Could you check a few things on this model? Use its own coordinates, in mm. A direction names the side the tool comes from. Coordinates: 2 decimals unless noted, no trailing zeros. Write each loop counter-clockwise with the first axis right and the second up, starting at its lowest first coordinate (ties: lowest second). Pieces come first, ordered by that corner, then holes. Notation, with made-up numbers: M -28,12.25 L -4,12.25 A12 ccw -4,16.25 Z; hole C 48,39.25 d11. An arc over 180 degrees is marked long. Answer as CSV lines item,"result". Start each with the question number.
Item 1: Suppose I cut it at B-B, the plane x = 0.25. Write out the boundary of the cut face in (y, z), and give its area (3 significant figures).
Item 2: We'd pull the mould along X, two halves only. Please class faces 5 (the flat face through (-2.74, -4, 3)), 6 (the flat face through (-6.584, -11, 4)), 7 (the flat face through (-9, -15, 2)), 8 (the flat face through (8.461, -4, 3)): +X half, -X half, draft (parallel to the pull), parting line (faces both ways), or undercut.
Item 3: On a 3-axis mill with a long thin cutter (end or side, diameter ignored), from which of +Z, -Z, +X, -X, +Y, -Y can I reach the whole of each face in a straight line? I mean faces 1 (the flat face through (3, -4, 4)), 2 (the flat face through (-9, -3.903, 5)), 3 (the flat face through (-9, -5.903, 4)), 4 (the flat face through (-2, -10.903, 1)). Say none if no direction works.
Item 4: Suppose I cut it at C-C, the plane z = 4.5. Write out the boundary of the cut face in (x, y), and give its area (3 significant figures).
Item 5: I'm going to push flat-ended pins straight in: P1, Ø7, axis at x = 2, y = -3, coming from the +Z side; P2, Ø1.6, axis at x = 5, z = 2.5, coming from the -Y side; P3, Ø2.5, axis at y = -13, z = 4.5, coming from the -X side. Where does each tip first touch, or does it pass through?
Item 6: Suppose I cut it at D-D, the plane x = -10. Write out the boundary of the cut face in (y, z).
Item 7: Suppose I cut it at A-A, the plane y = -12.25. Write out the boundary of the cut face in (x, z).
Item 8: If I drill on line 1 along Z through (x, y) = (7.25, -1); line 2 along Z through (x, y) = (-2.25, 1.75); line 3 along X through (y, z) = (-7.25, 5.25), over which ranges is the centre line in solid material (lowest first)? Write a range as [from, to].
```python
from build123d import *

# Parameters (mm, degrees)
SKETCH_2_W      = 25
SKETCH_2_H      = 15
EXTRUDE_1_DEPTH = 2
SKETCH_4_R      = 1.75
EXTRUDE_2_DEPTH = 7
SKETCH_5_W      = 5
SKETCH_5_H      = 5
EXTRUDE_3_DEPTH = 2
SKETCH_4_3_R    = 1.75
EXTRUDE_4_DEPTH = 2
SKETCH_7_W      = 11.201035141
SKETCH_7_H      = 8.645905099
EXTRUDE_5_DEPTH = 2
SKETCH_4_4_R    = 1.75
EXTRUDE_6_DEPTH = 8


with BuildPart() as part:
    # Sketch 2 → Extrude 1 (new body)
    with BuildSketch(Plane.XY):
        with Locations((-1.845610675, -3.40346801)):
            Rectangle(SKETCH_2_W, SKETCH_2_H)
    extrude(amount=EXTRUDE_1_DEPTH)

    # Sketch 4 → Extrude 2 (add)
    with BuildSketch(Plane.XZ.offset(10.90346801)):
        Polygon((-11.584222065, 7), (-11.584222065, 2), (-11.507000867, 2), (-6.584222065, 2), (-6.584222065, 7), align=None)
        with Locations((-9.064916765, 4.5)):
            Circle(SKETCH_4_R, mode=Mode.SUBTRACT)
    extrude(amount=-EXTRUDE_2_DEPTH)

    # Sketch 5 → Extrude 3 (add)
    with BuildSketch(Plane(origin=(0, -3.90346801, 0), x_dir=(1, 0, 0), z_dir=(0, 1, 0))):
        with Locations((-9.084222065, -4.5)):
            Rectangle(SKETCH_5_W, SKETCH_5_H)
    extrude(amount=-EXTRUDE_3_DEPTH)

    # Sketch 4_3 → Extrude 4 (add)
    with BuildSketch(Plane.XZ.offset(10.90346801)):
        Polygon((-11.584222065, 7), (-11.584222065, 2), (-11.507000867, 2), (-6.584222065, 2), (-6.584222065, 7), align=None)
        with Locations((-9.064916765, 4.5)):
            Circle(SKETCH_4_3_R, mode=Mode.SUBTRACT)
    extrude(amount=EXTRUDE_4_DEPTH)

    # Sketch 7 → Extrude 5 (add)
    with BuildSketch(Plane.XY.offset(2)):
        with Locations((2.86075116, -3.79430768)):
            Rectangle(SKETCH_7_W, SKETCH_7_H)
    extrude(amount=EXTRUDE_5_DEPTH)

    # Sketch 4_4 → Extrude 6 (add)
    with BuildSketch(Plane.XZ.offset(10.90346801)):
        Polygon((-11.584222065, 7), (-11.584222065, 2), (-11.507000867, 2), (-6.584222065, 2), (-6.584222065, 7), align=None)
        with Locations((-9.064916765, 4.5)):
            Circle(SKETCH_4_4_R, mode=Mode.SUBTRACT)
    extrude(amount=EXTRUDE_6_DEPTH)


solid = part.part
```
Ans:
1,outline,"M -10.9,0 L 4.1,0 L 4.1,2 L 0.53,2 L 0.53,4 L -8.12,4 L -8.12,2 L -10.9,2 Z"
1,area,"47.3 mm^2"
2,face 5,"undercut"
2,face 6,"undercut"
2,face 7,"draft"
2,face 8,"+X half"
3,face 1,"+Z, +X, +Y, -Y"
3,face 2,"+Z, -X, +Y"
3,face 3,"-Y"
3,face 4,"-Z, +X, -X, -Y"
4,outline,"M -11.58,-18.9 L -10.81,-18.9 L -10.81,-5.9 L -7.31,-5.9 L -7.31,-18.9 L -6.58,-18.9 L -6.58,-3.9 L -11.58,-3.9 Z"
4,area,"29.5 mm^2"
5,P1,"stops at z = 4"
5,P2,"stops at y = -10.9"
5,P3,"stops at x = -11.58"
6,outline,"M -18.9,2 L -10.9,2 L -10.9,0 L 4.1,0 L 4.1,2 L -3.9,2 L -3.9,7 L -18.9,7 L -18.9,5.98 L -5.9,5.98 L -5.9,3.02 L -18.9,3.02 Z"
7,outline,"M -11.58,2 L -6.58,2 L -6.58,7 L -11.58,7 Z; hole C -9.06,4.5 d3.5"
8,line 1,"z = [0, 4]"
8,line 2,"z = [0, 2]"
8,line 3,"x = [-11.58, -10.65], [-7.48, -6.58]"
